Input: dimensioned drawing with shaded views. Units: mm. Origin: part minimum x, y, z. Give positions to 0.01 mm unless a question says otherwise; leave off trailing zeros. Loops run counter-clockwise (first coordinate to the right, second up) from the corner with the lowest first, then second, coordinate; pieces in that order, holes last.
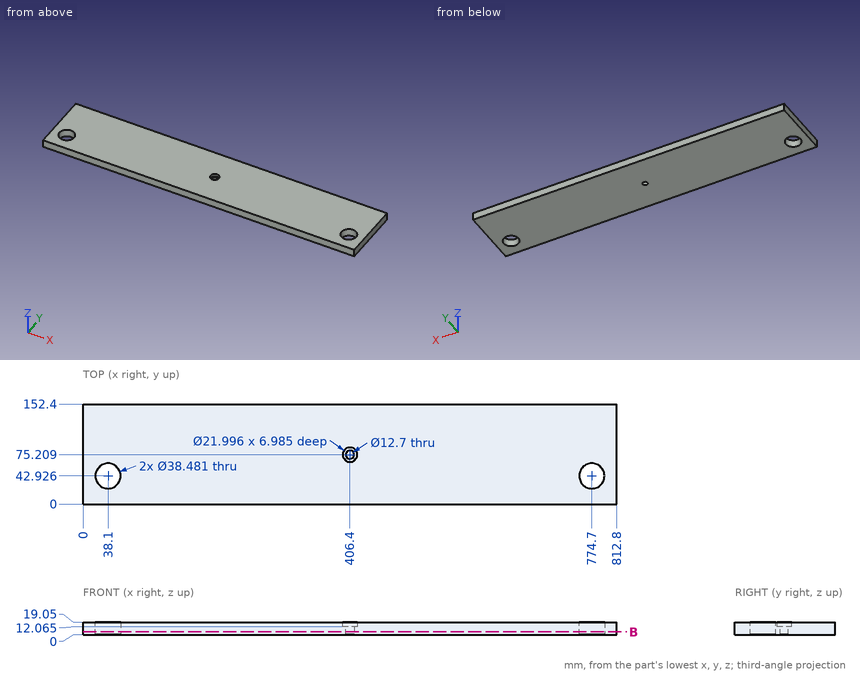
(1) Ray query, line 1 along X through (y, z) = (35, 4.5); line 2 along X through (y, z) = (27, 11) (1 decimal); line 3 along Y through (x, z) = (774.7, 6.5) (1 decimal). Return the intervals inside material, ascending.
A:
line 1: x = 0 to 20.57, 55.63 to 757.17, 792.23 to 812.8
line 2: x = 0 to 27.3, 48.9 to 763.9, 785.5 to 812.8
line 3: y = 0 to 23.7, 62.2 to 152.4
(2) First-contact query: pin 1 (11 mm diameter, centred on x = 408.5, y = 76.5, fed in from +Z) (3 decimals). Flat tip, straight axial feed; report the tip coordinate or a pass-through.
A:
pin 1: stops at z = 12.065
(3) Section B-B, the plane z = 4. Return the cut outline in (x, y).
A:
outline: (0, 0) - (812.8, 0) - (812.8, 152.4) - (0, 152.4) - close; hole circle Ø38.48 at (38.1, 42.93); hole circle Ø12.7 at (406.4, 75.21); hole circle Ø38.48 at (774.7, 42.93)
